Answer from the drawing. Dimensions are ordinates in mm from the lowest x, y and z of the part. A direction names the side the tool comes from. Give positions to 0.01 mm unless a question says otherwise; leave off trailing zeros. Loops run counter-clockwise (first coordinate to the right, second up) from the corner with the lowest first, then second, coordinate; pieces in that order, holes last. Notation, with made-up numbers: (39, -8.5) - (64, -8.5) arc R16 cw to (64, 12.5) - close; hole circle Ø11 at (3, 9.25). An arc over 180 degrees is marked (long way). Write each question's results on one line, items separated by ' | '. Start each with the question number.
Q1. The part is cut by section A-A, the plane x = 101.5. Write down the section's boundary in (y, z).
Q2. Determine the mould class of the marked faces 3, 4 and 5 for opening direction Y: +Y half, -Y half, draft (parallel to the pull), parting line (faces both ways), or undercut.
Q3. The part is cut by section C-C, the plane z = 103. Write down the section's boundary in (x, y), plus the area to 3 significant figures.
Q4. Given pin 1 (1 mm diameter, centred on y = 214.5, z = 53.5, fed in from -X), flat-ended and moving along its own axis, determine where the tip first touches the part or whether it passes through.
Q5. Find the intervals of material crossed by line 1 (X direction, y = 187, z = 98); line 2 (Y direction, x = 85.5, z = 168), in increasing order. Write a range as from..to.
Q6. For the marked faces 1 and 2, determine the directions among +Z, -Z, +X, -X, +Y, -Y from which every point of the face is accessible in a straight line to the end or side of a thin tool.
Q7. The part is cut by section B-B, the plane y = 510. Write down the section's boundary in (x, z).
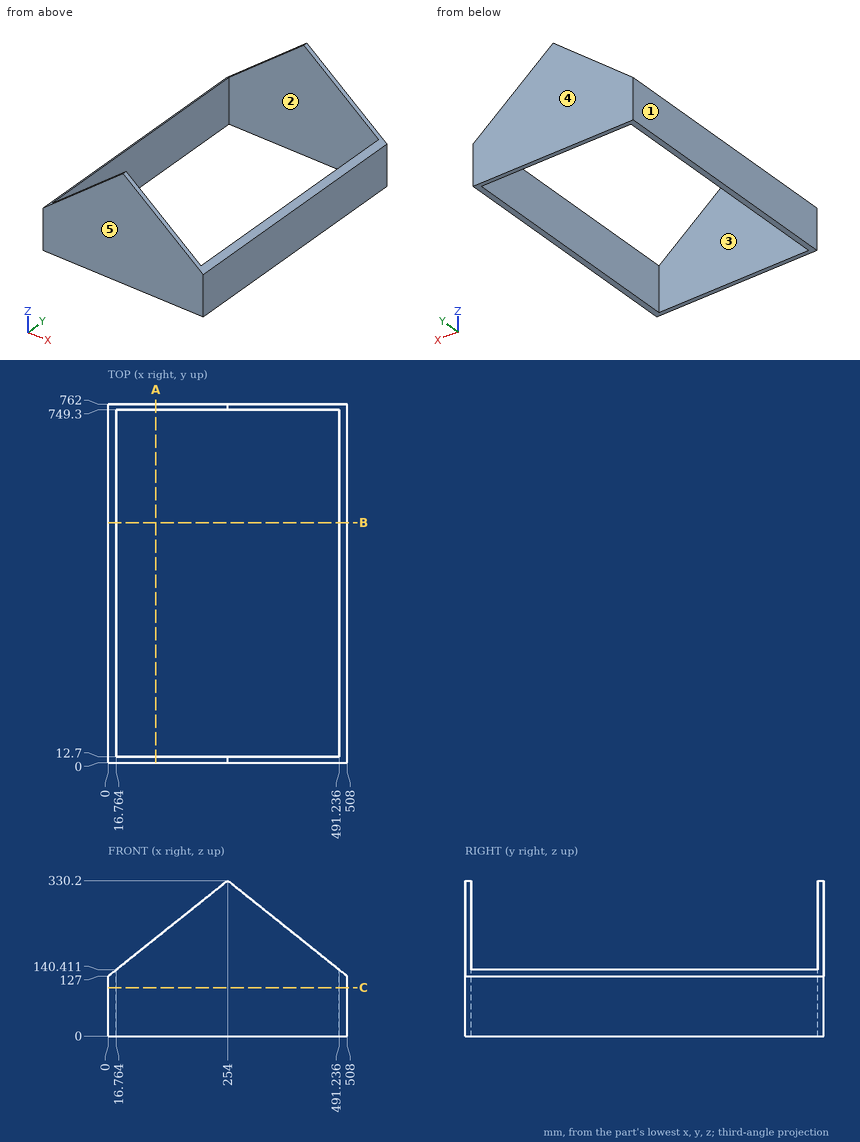
Check sheet entries:
1) outline: (0, 0) - (12.7, 0) - (12.7, 208.2) - (0, 208.2) - close; (749.3, 0) - (762, 0) - (762, 208.2) - (749.3, 208.2) - close
2) face 3: undercut | face 4: +Y half | face 5: -Y half
3) outline: (0, 0) - (508, 0) - (508, 762) - (0, 762) - close; hole (16.76, 12.7) - (491.24, 12.7) - (491.24, 749.3) - (16.76, 749.3) - close | area: 37,600 mm^2
4) pin 1: stops at x = 0
5) line 1: x = 0..16.76, 491.24..508 | line 2: y = 0..12.7, 749.3..762
6) face 1: +Z, -Z, -X, +Y, -Y | face 2: +Z, -Z
7) outline: (0, 0) - (16.76, 0) - (16.76, 140.41) - (0, 127) - close; (491.24, 0) - (508, 0) - (508, 127) - (491.24, 140.41) - close
